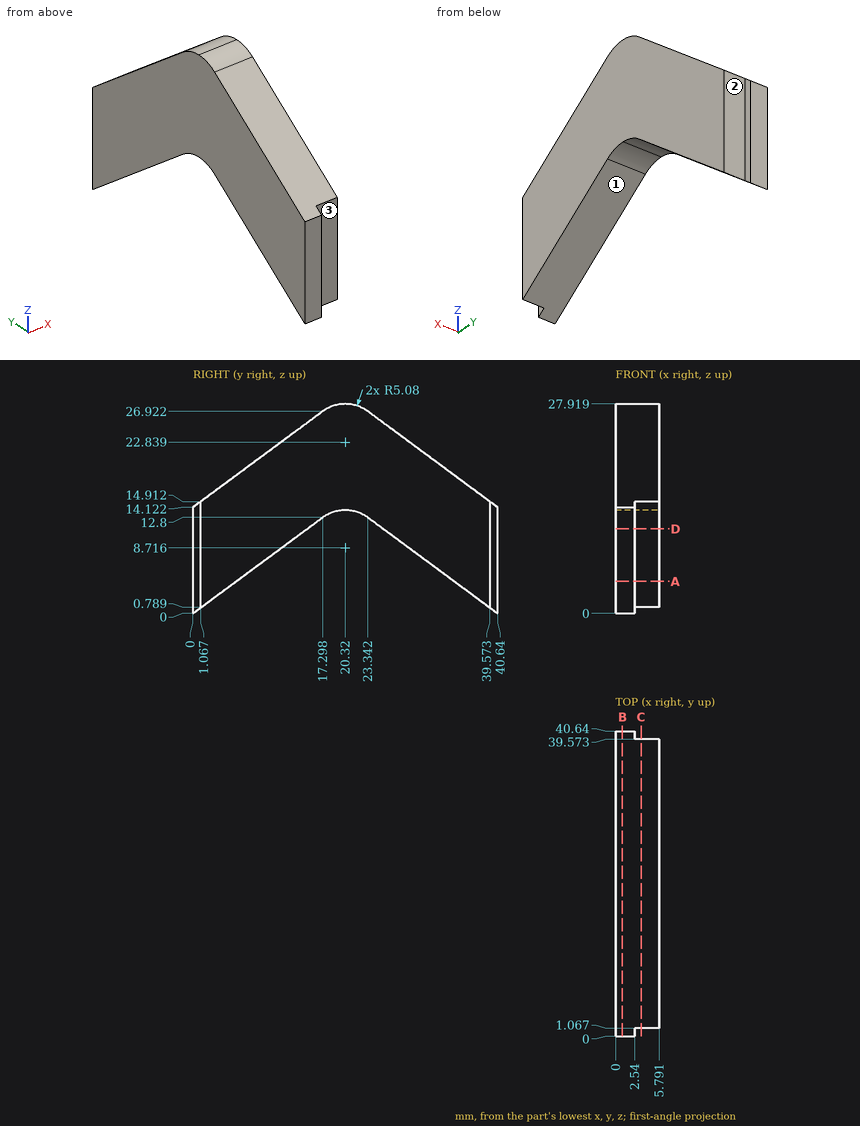
Source: three-view drawing plus pictorial views. Frame: mm from the lowest corner of the part. A direction names the side the tool comes from. Give positions to 0.01 mm unless a question says otherwise; leave off trailing zeros. Order: outer loops, then holes, each group sorted by start corner. A loop starts at its lowest first (then second) coordinate and runs counter-clockwise, first axis right, second up. Notation, with made-up numbers: M 80.5,80.5 L 112.5,80.5 A22 ccw 112.5,104.5 Z; hole C 64,-4 d2. An arc over 180 degrees is marked long. Return JSON: item names as keys, results as strings.
1) Section query B-B on x = 0.9. Output: boundary loops of the cut face in (y, z).
Taken from the geometry:
{"outline": "M 0,0 L 17.3,12.8 A5.08 cw 23.34,12.8 L 40.64,0 L 40.64,14.12 L 23.34,26.92 A5.08 ccw 17.3,26.92 L 0,14.12 Z"}
2) Line query: L1, parallel to Y at x = 2.8, z = 11.75 (1 decimal); L2, parallel to Y at x = 2.95, z = 8 (1 decimal); L3, parallel to Y at x = 1.5, z = 23.5 (1 decimal). Output: solid intervals per line, ascending. Write a range as [from, to].
Taken from the geometry:
{"L1": "y = [1.1, 15.9], [24.8, 39.6]", "L2": "y = [1.1, 10.8], [29.8, 39.6]", "L3": "y = [12.7, 28]"}
3) Contact query for flat-ended pins moving along their axis: pin 1 (1.5 mm diameter, centred on x = 1, y = 25.5, fed in from +Z); pin 2 (0.9 mm diameter, centred on y = 40.5, z = 6.5, fed in from +X); pin 3 (3 mm diameter, centred on x = 3, y = 31, fed in from +Z) (1 decimal). Output: stop coordinate, or through.
Taken from the geometry:
{"pin 1": "stops at z = 25.88", "pin 2": "stops at x = 2.54", "pin 3": "stops at z = 22.4"}
4) Access query for the marked faces 1, 2 and 3. Directions: +Z, -Z, +X, -X, +Y, -Y. A direction counts if a zero-diameter tool reaches every point of the face in a straight line with its end or side. Return the directions, or none.
Taken from the geometry:
{"face 1": "-Z, +X, -X", "face 2": "+Z, -Z, +X, +Y", "face 3": "+Z, -Z, +X, -Y"}
5) Section query C-C on x = 3.4. Output: boundary loops of the cut face in (y, z).
Taken from the geometry:
{"outline": "M 1.07,0.79 L 17.3,12.8 A5.08 cw 23.34,12.8 L 39.57,0.79 L 39.57,14.91 L 23.34,26.92 A5.08 ccw 17.3,26.92 L 1.07,14.91 Z"}
6) Section query D-D on z = 11.25. Output: boundary loops of the cut face in (x, y), and give its area (3 significant figures).
Taken from the geometry:
{"outline": "M 0,0 L 2.54,0 L 2.54,1.07 L 5.79,1.07 L 5.79,15.2 L 0,15.2 Z; M 0,25.44 L 5.79,25.44 L 5.79,39.57 L 2.54,39.57 L 2.54,40.64 L 0,40.64 Z", "area": "169 mm2"}
7) Section query A-A on z = 4.25. Output: boundary loops of the cut face in (x, y).
Taken from the geometry:
{"outline": "M 0,0 L 2.54,0 L 2.54,1.07 L 5.79,1.07 L 5.79,5.74 L 0,5.74 Z; M 0,34.9 L 5.79,34.9 L 5.79,39.57 L 2.54,39.57 L 2.54,40.64 L 0,40.64 Z"}
